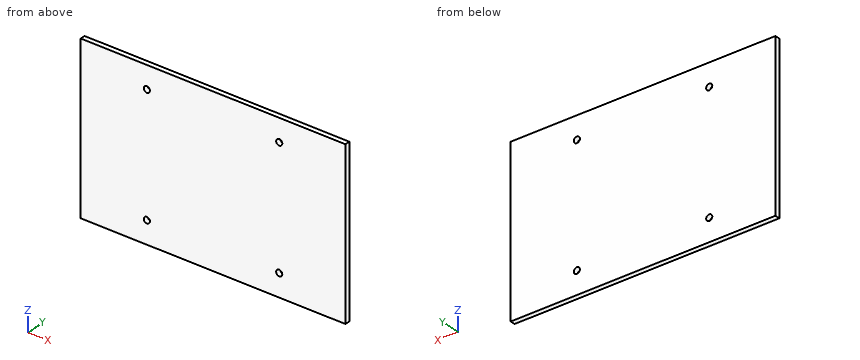
Autodesk Inventor part; units mm, degrees
ref_plane "YZ Plane" through (0, 0, 0) normal (1, 0, 0) x (0, 1, 0)
ref_plane "XZ Plane" through (0, 0, 0) normal (0, 1, 0) x (-1, 0, 0)
ref_plane "XY Plane" through (0, 0, 0) normal (0, 0, 1) x (1, 0, 0)
sketch "Эскиз1" plane through (0, 0, 0) normal (0, 1, 0) x (-1, 0, 0)
  circle A0 centre (-40, 85.5) radius 1.85
  circle A1 centre (-40, 13.5) radius 1.85
  circle A2 centre (-120, 85.5) radius 1.85
  circle A3 centre (-120, 13.5) radius 1.85
  line L0 (0, 99) -> (0, 68.3189)
  line L1 (0, 99) -> (-160, 99)
  line L2 (-160, 0) -> (0, 0)
  line L3 (-160, 30.6811) -> (-160, 0)
  line L4 (0, 99) -> (-160, 99)
  line L5 (-160, 99) -> (-160, 0)
  line L6 (-160, 0) -> (0, 0)
  line L7 (0, 0) -> (0, 99)
extrude "Выдавливание1" add sketch "Эскиз1" along normal blind 3
properties part number "KB33-046-004-001 - Центральная пластина" material "Дерево (вишня)"
Here's how the part is built. I have some questions about the finished solid (model axes, mm). Round coordinates to 2 decimals unless told otherwise and drop trailing zeros. Order: outer loops, then holes, each group sorted by start corner. A loop starts at its lowest first (then second) coordinate and runs counter-clockwise, first axis right, second up. Notation, with made-up numbers: M 68,32 L 111,32 A23 cw 111,52 Z; hole C 67.25,2.25 d2. An arc over 180 degrees is marked long. Answer as CSV lines item,"result".
Item 1: Imagine slicing it at A-A on z = 85.5. List the corners of the cut face in (x, y) for me.
From the geometry:
outline,"M 0,0 L 38.15,0 L 38.15,3 L 0,3 Z; M 41.85,0 L 118.15,0 L 118.15,3 L 41.85,3 Z; M 121.85,0 L 160,0 L 160,3 L 121.85,3 Z"
Item 2: Please list where these lines run through material, in increasing order: L1, parallel to X at y = 1.5, z = 85.5; L2, parallel to Z at x = 120, y = 1.9; L3, parallel to Z at x = 41.5, y = 1.3. Write a range as [from, to].
From the geometry:
L1,"[0, 38.15], [41.85, 118.15], [121.85, 160]"
L2,"[0, 11.65], [15.35, 83.65], [87.35, 99]"
L3,"[0, 12.42], [14.58, 84.42], [86.58, 99]"
Item 3: Imagine slicing it at B-B on x = 120. List the corners of the cut face in (y, z) for me, and give its area (3 significant figures).
From the geometry:
outline,"M 0,0 L 3,0 L 3,11.65 L 0,11.65 Z; M 0,15.35 L 3,15.35 L 3,83.65 L 0,83.65 Z; M 0,87.35 L 3,87.35 L 3,99 L 0,99 Z"
area,"275 mm2"
